Check sheet for the drawn part. Datum: minimum x, y, z corner. Units: mm. A direction names the side the tool comes from. Coordinates: 2 decimals unless noted, no trailing zeros. Order: outer loops, then holes, each group sorted by start corner. A loop starts at its lowest first (then second) coordinate and runs counter-clockwise, first axis right, second up. Notation, with made-up numbers: (-7, 57) - (38, 57) arc R10 ccw to (38, 69) - close; hole circle Ø7 at (45, 75). An arc over 180 degrees is marked (long way). Return JSON: item names as keys, results as strings. Group by question number.
Item 1: Section check D-D on x = 8.5. Enter the section's corners in (y, z) (3 decimals), then the cut area to 3 significant figures.
Item 2: Gauge pin test, flat ends, axial feed: pin 1 (3 mm diameter, centred on x = 28, y = 3.5, fed in from +Z); pin 2 (8 mm diameter, centred on x = 18.5, z = 25.5, fed in from +Y); pin 3 (1.5 mm diameter, centred on x = 6, y = 1.5, fed in from +Z); pin 4 (10 mm diameter, centred on x = 16.51, z = 16.51, fed in from +Y) (3 decimals). Record the tip position at first contact, or that the pin passes through.
Item 3: Tool access check on the marked faces 4 and 5. Record the directions out of +Z, -Z, +X, -X, +Y, -Y that give a thin tool (end or side, any length) a straight path to the whole face; none if there is none.
Item 4: Scan lines: probe 1 along Z at (x, y) = (17, 6.75); probe 2 along X at (y, z) = (3.6, 16.51); probe 3 along Z at (x, y) = (16.51, 1.2). Record each from-to range of solid material in increasing order.
Item 5: Section check C-C on y = 4. Enter the section's corners in (x, z).
Item 6: Section check A-A on x = 16.51. Enter the section's corners in (y, z) (3 decimals), then the cut area to 3 significant figures.
Item 7: Section check B-B on z = 16.51. Enter the section's corners in (x, y) (3 decimals).
Item 8: Draft check along Z on the marked faces 1, 2 and 3. Enter one of: pulls with the +Z half, pulls with the -Z half, needs draft (parallel to the pull), parting line crosses it, or undercut.
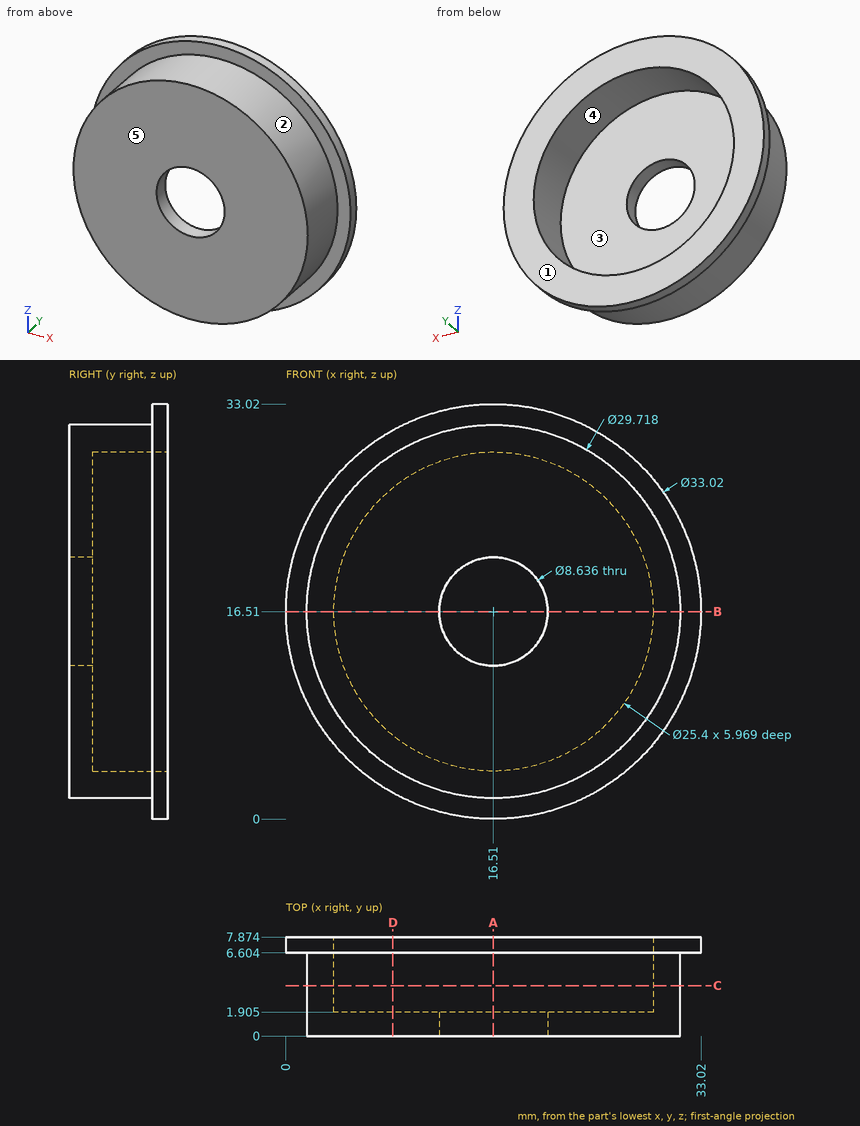
Computed:
{
 "1": {"outline": "(0, 3.995) - (6.604, 3.995) - (6.604, 2.073) - (7.874, 2.073) - (7.874, 6.655) - (1.905, 6.655) - (1.905, 26.365) - (7.874, 26.365) - (7.874, 30.947) - (6.604, 30.947) - (6.604, 29.025) - (0, 29.025) - close", "area": "84.3 mm²"},
 "2": {"pin 1": "stops at z = 27.51", "pin 2": "stops at y = 7.87", "pin 3": "stops at z = 27.71", "pin 4": "stops at y = 1.905"},
 "3": {"face 4": "+Y", "face 5": "+Z, -Z, +X, -X, -Y"},
 "4": {"probe 1": "z = 0.01 to 3.82, 29.2 to 33.01", "probe 2": "x = 1.65 to 3.81, 29.21 to 31.37", "probe 3": "z = 1.65 to 12.19, 20.83 to 31.37"},
 "5": {"outline": "circle Ø29.72 at (16.51, 16.51); hole circle Ø25.4 at (16.51, 16.51)"},
 "6": {"outline": "(0, 1.651) - (6.604, 1.651) - (6.604, 0) - (7.874, 0) - (7.874, 3.81) - (1.905, 3.81) - (1.905, 12.192) - (0, 12.192) - close; (0, 20.828) - (1.905, 20.828) - (1.905, 29.21) - (7.874, 29.21) - (7.874, 33.02) - (6.604, 33.02) - (6.604, 31.369) - (0, 31.369) - close", "area": "70.1 mm²"},
 "7": {"outline": "(0, 6.604) - (1.651, 6.604) - (1.651, 0) - (12.192, 0) - (12.192, 1.905) - (3.81, 1.905) - (3.81, 7.874) - (0, 7.874) - close; (20.828, 0) - (31.369, 0) - (31.369, 6.604) - (33.02, 6.604) - (33.02, 7.874) - (29.21, 7.874) - (29.21, 1.905) - (20.828, 1.905) - close"},
 "8": {"face 1": "needs draft", "face 2": "parting line crosses it", "face 3": "undercut"}
}
